Autodesk Inventor part; units mm, degrees
ref_plane "Work Plane1" through (431.8, 0, 0) normal (1, 0, 0) x (0, 1, 0)
ref_plane "Work Plane2" through (-25.4, 0, 0) normal (1, 0, 0) x (0, 1, 0)
ref_plane "Work Plane3" through (203.2, 0, 0) normal (1, 0, 0) x (0, 1, 0)
sketch "Sketch1" plane through (0, 0, 0) normal (0, 0, 1) x (1, 0, 0)
  line L0 (0, 25.4) -> (406.4, 25.4)
  line L1 (406.4, 25.4) -> (406.4, -25.4)
  line L2 (406.4, -25.4) -> (0, -25.4)
  line L3 (0, -25.4) -> (0, 25.4)
  circle A0 centre (0, 0) radius 25.4
  circle A1 centre (406.4, 0) radius 25.4
  dimension "d0" = 406.4
  dimension "d1" = 50.8
extrude "Extrusion1" add sketch "Sketch1" along normal mid plane 50.8
sketch "Sketch2" plane through (0, 25.4, 25.4) normal (0, 1, 0) x (1, 0, 0)
  line L0 (-25.4, 50.8) -> (-25.4, 0)
  line L1 (-25.4, 50.8) -> (0, 50.8)
  line L2 (0, 0) -> (-25.4, 0)
  line L3 (0, 0) -> (406.4, 0)
  line L4 (406.4, 50.8) -> (0, 50.8)
  line L5 (-25.4, 12.7) -> (25.4, 12.7)
  line L6 (25.4, 12.7) -> (25.4, 38.1)
  line L7 (25.4, 38.1) -> (-25.4, 38.1)
  line L8 (-25.4, 38.1) -> (-25.4, 12.7)
  point P0 (-25.4, 25.4)
  point P1 (-25.4, 25.4)
  dimension "d4" = 25.4
  dimension "d10" = 50.8
extrude "Extrusion2" cut sketch "Sketch2" against normal through all
ref_plane "Work Plane1" through (431.8, 0, 0) normal (1, 0, 0) x (0, 1, 0)
ref_plane "Work Plane2" through (-25.4, 0, 0) normal (1, 0, 0) x (0, 1, 0)
ref_plane "Work Plane3" through (203.2, 0, 0) normal (1, 0, 0) x (0, 1, 0)
sketch "Sketch5" plane through (0, 0, 25.4) normal (0, 0, 1) x (1, 0, 0)
  arc A0 (406.4, -25.4) -> (406.4, 25.4) centre (406.4, 0) ccw
  line L0 (0, 25.4) -> (406.4, 25.4)
  arc A1 (0, 25.4) -> (0, -25.4) centre (0, 0) ccw
  line L1 (406.4, -25.4) -> (0, -25.4)
  circle A2 centre (0, 0) radius 25.4 construction
  circle A3 centre (406.4, 0) radius 25.4 construction
  line L2 (38.1, 25.4) -> (38.1, -25.4)
  line L3 (368.3, 25.4) -> (368.3, -25.4)
  dimension "d11" = 12.7
  dimension "d13" = 12.7
extrude "Extrusion4" cut sketch "Sketch5" against normal blind 3.175 contours L1 L2 L0 L3
pattern_circular "Circular Pattern1" count 4 over 360 about axis through (-10, 0, 0) along (1, 0, 0) of "Extrusion4"
mirror "Mirror1" about plane through (203.2, 0, 0) normal (1, 0, 0) of "Extrusion2"
sketch "Sketch3" plane through (0, 0, 25.4) normal (0, 0, 1) x (1, 0, 0)
  arc A0 (0, 25.4) -> (0, -25.4) centre (0, 0) ccw
  arc A1 (406.4, -25.4) -> (406.4, 25.4) centre (406.4, 0) ccw
  circle A2 centre (0, 0) radius 12.7
  circle A3 centre (406.4, 0) radius 12.7
  dimension "d7" = 25.4
extrude "Extrusion3" add sketch "Sketch3" along normal blind 3.175
mirror "Mirror2" about plane through (0, 0, 0) normal (0, 0, 1) of "Extrusion3"
equation "\"d13\" = d11"
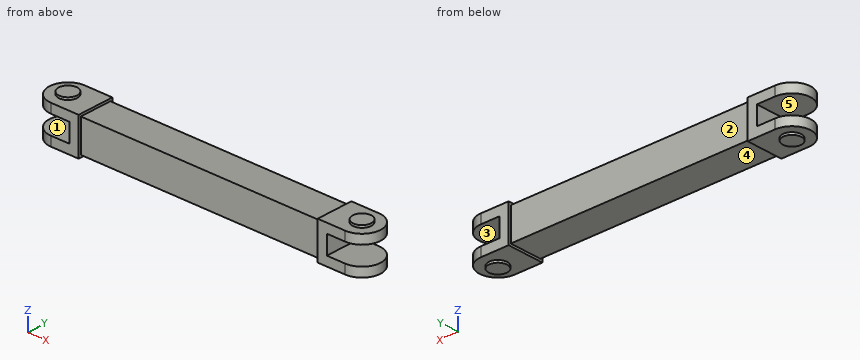
Could you check a few things on this model? Use its own coordinates, in mm. Face numbers are marked on the shaded views. A direction names the side the tool comes from. Give positions to 0.01 mm unless a question says otherwise; leave off trailing zeros. Order: outer loops, then holes, each group sorted by start corner. A loop starts at its lowest first (then second) coordinate and runs counter-clockwise, first axis right, second up. Notation, with made-up numbers: (1.25, 63) - (49.25, 63) arc R29 cw to (49.25, 97) - close; hole circle Ø3 at (77, -40). An arc over 180 degrees is marked (long way). One line per item, written item: value. Start each with the question number.
1. Imagine slicing it at A-A on z = -4. List the corners of the cut face in (x, y) for me (3 decimals).
2. Imagine slicing it at B-B on x = 229.5. List the corners of the cut face in (y, z) for me (3 decimals), plus the area to 3 significant figures.
3. If I drill on probe 1 along Z at (x, y) = (-5, 4.5) (3 decimals); probe 2 along Y at (x, z) = (208, 15) (3 decimals); probe 3 along X at (y, z) = (17.5, 1.5), over which ranges is the centre line in solid material (lowest first)?
4. For P1, Ø3, axis at y = 8.5, z = 12.5, coming from the -X side; P2, Ø3, axis at x = 341, y = 14, coming from the -Z side (3 decimals); P3, Ø8, axis at y = -10.5, z = 14, coming from the +X side, each with a flat end and sliding along its axis, tell me the tip position at first contact or that it passes through.
5. For the marked faces 1, 2 and 3, which set-ups out of +Z, -Z, +X, -X, +Y, -Y let a thin tool reach every point of the face, with its end or its side?
6. Thinking about a two-plate mould opening in X: for the marked faces 4 and 5, which applies, +X half, -X half, draft (parallel to the pull), parting line (faces both ways), or undercut?
Values:
1. outline: (25.4, -25.4) - (38.1, -25.4) - (38.1, -22.225) - (368.3, -22.225) - (368.3, -25.4) - (381, -25.4) - (381, 25.4) - (368.3, 25.4) - (368.3, 22.225) - (38.1, 22.225) - (38.1, 25.4) - (25.4, 25.4) - close
2. outline: (-22.225, -22.225) - (22.225, -22.225) - (22.225, 22.225) - (-22.225, 22.225) - close
2. area: 1,980 mm²
3. probe 1: -28.575 to -12.7, 12.7 to 28.575
3. probe 2: -22.225 to 22.225
3. probe 3: 25.4 to 381
4. P1: x = -24.41
4. P2: z = -22.225
4. P3: x = 430.95
5. face 1: -X, +Y, -Y
5. face 2: +Z, -Z, +Y
5. face 3: +X, +Y, -Y
6. face 4: undercut
6. face 5: draft
